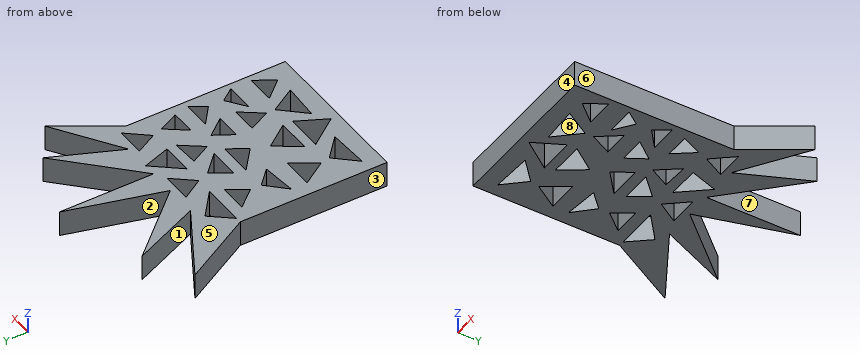
```python
from build123d import *

# Parameters (mm, degrees)
F1_DEPTH = 7


with BuildPart() as f1:
    # F0 (on Top) → F1 (new body)
    with BuildSketch(Plane.XY):
        Polygon((-34.109668, 24.133805), (-34.109668, -15.859125), (9.286875, -15.859125), (9.286875, 27.439939), (9.286875, 27.574874), (19.288125, 43.291125), (1.894246, 31.575374), (9.858374, 49.863376), (-8.715375, 31.575374), (-8.715375, 57.292875), (-15.873495, 31.575374), (-32.432627, 49.863376), (-24.468496, 31.575374), (-44.719875, 43.291125), align=None)
        Polygon((-19.780688, -10.786669), (-30.718125, -11.287125), (-25.574625, -5.572125), align=None, mode=Mode.SUBTRACT)
        Polygon((-13.858875, -13.573125), (-19.780688, -5.572125), (-9.858374, -5.572125), align=None, mode=Mode.SUBTRACT)
        Polygon((-26.146125, -3.000375), (-30.432375, 3.571875), (-21.859875, 3.571875), align=None, mode=Mode.SUBTRACT)
        Polygon((-9.858374, -3.000375), (-19.002376, -3.000375), (-14.716125, 3.571875), align=None, mode=Mode.SUBTRACT)
        Polygon((-21.233711, 8.792836), (-30.432375, 7.858125), (-25.479374, 12.934948), align=None, mode=Mode.SUBTRACT)
        Polygon((-12.873181, 7.858125), (-19.002376, 12.934948), (-9.936156, 12.934948), align=None, mode=Mode.SUBTRACT)
        Polygon((-25.479374, 15.859125), (-29.804411, 20.95796), (-22.234662, 20.95796), align=None, mode=Mode.SUBTRACT)
        Polygon((-9.936156, 15.859125), (-18.407172, 15.859125), (-15.162459, 20.95796), align=None, mode=Mode.SUBTRACT)
        Polygon((0, -11.287125), (-9.858374, -10.786669), (-4.143375, -4.43667), align=None, mode=Mode.SUBTRACT)
        Polygon((-4.143375, -2.143125), (-7.000875, 3.571875), (0, 3.571875), align=None, mode=Mode.SUBTRACT)
        Polygon((7.732536, -5.572125), (4.593785, -10.786669), (0, -5.572125), align=None, mode=Mode.SUBTRACT)
        Polygon((7.732536, 0), (0, 0), (5.000625, 3.696115), align=None, mode=Mode.SUBTRACT)
        Polygon((0, 7.858125), (-7.000875, 7.858125), (-4.06385, 12.934948), align=None, mode=Mode.SUBTRACT)
        Polygon((-7.000875, 15.859125), (-9.858374, 21.288376), (-2.783154, 21.583176), align=None, mode=Mode.SUBTRACT)
        Polygon((5.000625, 7.858125), (0, 11.858624), (7.732536, 11.858624), align=None, mode=Mode.SUBTRACT)
        Polygon((6.643688, 15.859125), (0, 15.859125), (4.0005, 21.288376), align=None, mode=Mode.SUBTRACT)
        Polygon((-20.936942, 24.133805), (-32.638886, 24.133805), (-27.985641, 29.860875), align=None, mode=Mode.SUBTRACT)
        Polygon((-16.371781, 24.133805), (-19.928829, 29.860875), (-11.718535, 29.860875), align=None, mode=Mode.SUBTRACT)
        Polygon((-2.783154, 24.133805), (-11.332653, 24.133805), (-5.286376, 31.575374), align=None, mode=Mode.SUBTRACT)
        Polygon((3.02262, 24.133805), (0, 29.860875), (7.732536, 29.860875), align=None, mode=Mode.SUBTRACT)
    extrude(amount=F1_DEPTH)


solid = f1.part
```
The model under review builds one solid part; all positions refer to its coordinate system, in mm. Face numbers are marked on the shaded views. A direction names the side the tool comes from. Coordinates: 2 decimals unless noted, no trailing zeros. Order: outer loops, then holes, each group sorted by start corner. A loop starts at its lowest first (then second) coordinate and runs counter-clockwise, first axis right, second up. Notation, with made-up numbers: (31, 40.5) -> (37, 40.5) arc R23 cw to (37, 72.5) -> close; hole circle Ø5 at (12.5, 11.5). An arc over 180 degrees is marked (long way). Answer in a Markdown table with one row per item. Add a question column.
Item 1: Clearance check with flat-ended pins moving along their axes: pin 1 (2 mm diameter, centred on x = -2, z = 2, fed in from +Y); pin 2 (2 mm diameter, centred on x = -7.5, z = 4, fed in from +Y); pin 3 (2 mm diameter, centred on x = -24, z = 3, fed in from +Y). State where each tip first meets the part, or that it passes through.
Item 2: To check wall thickness, follow probe 1 along X at (y, z) = (25, 2.25); probe 2 along Y at (x, z) = (-32, 4.5); probe 3 along Y at (x, z) = (7, 1.5). State the ranges of each line that lie inside material, in increasing order.
Item 3: We need section A-A on y = 45.5. Write out the cut boundary in (x, z).
Item 4: We need section C-C on z = 5. Give the number of separate pieces and of enclosed holes in the cut face, plus the area to 3 significant figures.
Item 5: We need section B-B on y = -1. Write out the cut boundary in (x, z), plus the area to 3 significant figures.
Item 6: Machinability: for the marked faces 5, 6, 7 and 8, which of the approach directions +Z, -Z, +X, -X, +Y, -Y give a long, thin tool a straight path to every point of the face, cutting with its end or side? Answer none if there is none.
Item 7: We need section D-D on y = 34. Write out the cut boundary in (x, z).
Item 8: Mouldability with a two-part tool opening along Y and no side actions: class the marked faces 1, 2, 3 and 4 as +Y half, -Y half, draft (parallel to the pull), parting line (faces both ways), or undercut.
Final values:
| question | item | result |
|---|---|---|
| 1 | pin 1 | stops at y = 39.17 |
| 1 | pin 2 | stops at y = 33.76 |
| 1 | pin 3 | stops at y = 41.65 |
| 2 | probe 1 | x = -34.59 to -31.94, -22 to -16.91, -15.67 to -10.63, -3.07 to 2.57, 3.73 to 9.29 |
| 2 | probe 2 | y = -15.86 to 24.13, 24.92 to 35.93, 48.87 to 49.39 |
| 2 | probe 3 | y = -15.86 to -6.79, -5.57 to 0, 0.99 to 10.79, 11.86 to 28.97, 29.86 to 35.01, 43.3 to 47.05 |
| 3 | outline | (-30.53, 0) -> (-28.48, 0) -> (-28.48, 7) -> (-30.53, 7) -> close; (-12, 0) -> (-8.72, 0) -> (-8.72, 7) -> (-12, 7) -> close; (5.43, 0) -> (7.96, 0) -> (7.96, 7) -> (5.43, 7) -> close |
| 4 | separate pieces | 1 |
| 4 | enclosed holes | 20 |
| 4 | area | 2,000 mm2 |
| 5 | outline | (-34.11, 0) -> (-27.45, 0) -> (-27.45, 7) -> (-34.11, 7) -> close; (-24.84, 0) -> (-17.7, 0) -> (-17.7, 7) -> (-24.84, 7) -> close; (-11.34, 0) -> (-4.71, 0) -> (-4.71, 7) -> (-11.34, 7) -> close; (-3.31, 0) -> (9.29, 0) -> (9.29, 7) -> (-3.31, 7) -> close |
| 5 | area | 231 mm2 |
| 6 | face 5 | +Z, +X, -X, +Y, -Y |
| 6 | face 6 | +Z, -Z, +X, -Y |
| 6 | face 7 | +Z, -Z, +Y |
| 6 | face 8 | +Z, -Z |
| 7 | outline | (-39.57, 0) -> (-28.66, 0) -> (-28.66, 7) -> (-39.57, 7) -> close; (-25.52, 0) -> (-18.07, 0) -> (-18.07, 7) -> (-25.52, 7) -> close; (-15.2, 0) -> (-8.72, 0) -> (-8.72, 7) -> (-15.2, 7) -> close; (-6.25, 0) -> (2.95, 0) -> (2.95, 7) -> (-6.25, 7) -> close; (5.49, 0) -> (13.38, 0) -> (13.38, 7) -> (5.49, 7) -> close |
| 8 | face 1 | undercut |
| 8 | face 2 | +Y half |
| 8 | face 3 | draft |
| 8 | face 4 | -Y half |
